Check sheet for the modelled part. Datum: model origin and axes. Units: mm. Round coordinates to 2 decimals unless told otherwise and drop trailing zeros. Write each loop counter-clockwise with the first axis right and the second up, starting at its lowest first coordinate (ties: lowest second). Pieces come first, ordered by that corner, then holes.
Item 1: Section check B-B, the plane y = -78. Record the cut outline in (x, z), plus the area to 3 significant figures.
Item 2: Depth check by flat-ended pin: pin 1 (2 mm diameter, centred on y = 93, z = 2, fed in from -X); pin 2 (1 mm diameter, centred on x = 156, z = 3, fed in from +Y); pin 3 (7.5 mm diameter, centred on x = -263.51, y = 198.99, fed in from -Z); pin 4 (5.5 mm diameter, centred on x = -173.83, y = 280.74, fed in from -Z). Enter the tip coordinate at first touch or a pass-through.
Item 3: Material ranges on line 1 along Y through (x, z) = (0, 1.5) (3 decimals); line 2 along Y through (x, z) = (-224.5, 2.5); line 3 along X through (y, z) = (-309.5, 2.5), recorded low to high.
Item 4: Section check C-C, the plane x = -105.5. Record the cut outline in (y, z).
Item 5: Section check A-A, the plane z = 4.5. State how many separate pieces and enclosed holes the cut face has, plus the area to 3 significant figures.
Autodesk Inventor part; units mm, degrees
ref_plane "YZ Plane" through (0, 0, 0) normal (1, 0, 0) x (0, 1, 0)
ref_plane "XZ Plane" through (0, 0, 0) normal (0, 1, 0) x (-1, 0, 0)
ref_plane "XY Plane" through (0, 0, 0) normal (0, 0, 1) x (1, 0, 0)
sketch "Sketch1" plane through (0, 0, 0) normal (0, 0, 1) x (1, 0, 0)
  circle A0 centre (0, 0) radius 355.6
  circle A1 centre (0, -330.2) radius 3.175
  circle A2 centre (119.282, -307.9023) radius 3.175
  circle A3 centre (222.4543, -244.0207) radius 3.175
  circle A4 centre (295.5829, -147.1828) radius 3.175
  circle A5 centre (328.7914, -30.467) radius 3.175
  circle A6 centre (317.5948, 90.3635) radius 3.175
  circle A7 centre (263.5053, 198.99) radius 3.175
  circle A8 centre (173.8279, 280.7417) radius 3.175
  circle A9 centre (60.6741, 324.5777) radius 3.175
  circle A10 centre (-60.6741, 324.5777) radius 3.175
  circle A11 centre (-173.8279, 280.7417) radius 3.175
  circle A12 centre (-263.5053, 198.99) radius 3.175
  circle A13 centre (-317.5948, 90.3635) radius 3.175
  circle A14 centre (-328.7914, -30.467) radius 3.175
  circle A15 centre (-295.5829, -147.1828) radius 3.175
  circle A16 centre (-222.4543, -244.0207) radius 3.175
  circle A17 centre (-119.282, -307.9023) radius 3.175
  line L0 (0, -342.9) -> (12.7, -342.9)
  line L1 (12.7, -342.9) -> (12.7, -349.25)
  line L2 (12.7, -349.25) -> (-12.7, -349.25)
  line L3 (-12.7, -349.25) -> (-12.7, -342.9)
  line L4 (-12.7, -342.9) -> (0, -342.9)
  line L5 (-75.5018, 334.7255) -> (-76.6688, 340.9674)
  line L6 (-63.0181, 337.0595) -> (-75.5018, 334.7255)
  line L7 (-50.5344, 339.3935) -> (-63.0181, 337.0595)
  line L8 (-76.6688, 340.9674) -> (-51.7014, 345.6354)
  line L9 (-51.7014, 345.6354) -> (-50.5344, 339.3935)
  dimension "d0" = 711.2
  dimension "d2" = 6.35
  dimension "d5" = 360
  dimension "d7" = 12.7
  dimension "d8" = 6.35
  dimension "d9" = 25.4
extrude "Extrusion1" add sketch "Sketch1" along normal blind 6.35
properties part number "laser circle3d back"
Values found:
1. outline: (-346.94, 0) - (346.94, 0) - (346.94, 6.35) - (-346.94, 6.35) - close
1. area: 4,410 mm2
2. pin 1: stops at x = -343.49
2. pin 2: stops at y = 319.8
2. pin 3: stops at z = 0
2. pin 4: passes through
3. line 1: y = -355.6 to -349.25, -342.9 to -333.375, -327.025 to 355.6
3. line 2: y = -275.77 to -246.45, -241.59 to 275.77
3. line 3: x = -175.1 to -122.03, -116.54 to 116.54, 122.03 to 175.1
4. outline: (-339.59, 0) - (339.59, 0) - (339.59, 6.35) - (-339.59, 6.35) - close
5. separate pieces: 1
5. enclosed holes: 19
5. area: 396,000 mm2
